The listing builds one solid part. Answer for the finished solid, in the listing's coordinates (mm). Give positions to 0.01 mm unless a question says otherwise; leave off trailing zeros. Order: outer loops, then holes, each group sorted by start corner. A loop starts at its lowest first (then second) coordinate and runs counter-clockwise, first axis right, second up. Notation, with made-up numbers: (-9, 1.25) - (4, 1.25) arc R9 ccw to (4, 12.25) - close; hole circle Ø6 at (-15.75, 16.25). An arc over 180 degrees is marked (long way). Answer as CSV lines item,"result". Start each with the question number.
1. Section C-C on z = 1.1 is taken. Give the vertices of the cut face in (x, y), and give its area (3 significant figures).
2. Consider line 1 along X through (y, z) = (0, 1.65); line 2 along Y through (x, z) = (2, 0.25); line 3 along X through (y, z) = (2.25, 0.65). Determine where each line is inside the solid, lowest interval first. Write a range as [from, to].
3. Section A-A on x = 2.5 is taken. Give the vertices of the cut face in (y, z), and give its area (3 significant figures).
4. A flat-ended cylindrical pin translates along its axis: pin 1 (1 mm diameter, centred on x = 4.5, z = 0.5, fed in from -Y). Find the tip coordinate at first contact, or state that the pin passes through.
5. Section D-D on y = -5 is taken. Give the vertices of the cut face in (x, z), and give its area (3 significant figures).
6. Section B-B on y = 2 is taken. Give the vertices of the cut face in (x, z), and give its area (3 significant figures).
7. Determine the mould class of faces 1 (the flat face through (-4.4, -1.3, 0)), 2 (the flat face through (-0.6, 5.29, 1.06)) for opening direction X: +X half, -X half, draft (parallel to the pull), parting line (faces both ways), or undercut.
from build123d import *

# Parameters (mm, degrees)
SKETCH_1_R          = 6.44
SKETCH_1_R_2        = 4.34
EXTRUDE_1_DEPTH     = 2.1
CUT_EXTRUDE_1_DEPTH = 7.44


with BuildPart() as part:
    # 草图1 → 凸台-拉伸1 (new body)
    with BuildSketch(Plane.XY):
        Circle(SKETCH_1_R)
        Circle(SKETCH_1_R_2, mode=Mode.SUBTRACT)
    extrude(amount=EXTRUDE_1_DEPTH)

    # 草图2 → 切除-拉伸1 (cut, through all)
    with BuildSketch(Plane(origin=(0, 0, 0), x_dir=(1, 0, 0), z_dir=(0, 1, 0))):
        Polygon((0, 0), (1.212435565, -2.1), (0, -2.1), (-1.212435565, 0), align=None)
    extrude(amount=CUT_EXTRUDE_1_DEPTH, mode=Mode.SUBTRACT)


solid = part.part
Checks:
1,outline,"(-0.58, 4.3) - (-0.58, 6.41) arc R6.44 ccw (long way) to (0.64, 6.41) - (0.64, 4.29) arc R4.34 cw (long way) to start"
1,area,"68.6 mm²"
2,line 1,"x = [-6.44, -4.34], [4.34, 6.44]"
2,line 2,"y = [-6.12, -3.85], [3.85, 6.12]"
2,line 3,"x = [-6.03, -3.71], [3.71, 6.03]"
3,outline,"(-5.93, 0) - (-3.55, 0) - (-3.55, 2.1) - (-5.93, 2.1) - close; (3.55, 0) - (5.93, 0) - (5.93, 2.1) - (3.55, 2.1) - close"
3,area,"10.0 mm²"
4,pin 1,"stops at y = -5.05"
5,outline,"(-4.06, 0) - (4.06, 0) - (4.06, 2.1) - (-4.06, 2.1) - close"
5,area,"17.0 mm²"
6,outline,"(-6.12, 0) - (-3.85, 0) - (-3.85, 2.1) - (-6.12, 2.1) - close; (3.85, 0) - (6.12, 0) - (6.12, 2.1) - (3.85, 2.1) - close"
6,area,"9.53 mm²"
7,face 1,"draft"
7,face 2,"undercut"
